```python
from build123d import *

# Parameters (mm, degrees)
SKETCH1_W              = 20
SKETCH1_H              = 35
SKETCH1_R              = 5
SKETCH1_R_2            = 1.1
BOSS_EXTRUDE1_DEPTH    = 13
SKETCH5_W              = 16
SKETCH5_H              = 31
CUT_EXTRUDE1_DEPTH     = 11
CUT_EXTRUDE2_REACH     = 40.652
SKETCH7_R              = 1.5
BOSS_EXTRUDE3_DEPTH    = 13
SKETCH11_R             = 3.25
CUT_EXTRUDE4_DEPTH     = 12
CUT_EXTRUDE5_START     = 12
CUT_EXTRUDE5_OUTLINE_R = 1.75
CUT_EXTRUDE5_DEPTH     = 1


# Read off the part's stored shape, not the designer's step: Cut-Extrude5
with BuildPart() as part:
    # Sketch1 → Boss-Extrude1 (new body)
    with BuildSketch(Plane(origin=(0, 0, 0), x_dir=(1, 0, 0), z_dir=(0, 1, 0))):
        with Locations((0, -7.840328725)):
            Rectangle(SKETCH1_W, SKETCH1_H)
        with Locations(Location((0, 0, 0), (0, 0, 90))):
            Circle(SKETCH1_R, mode=Mode.SUBTRACT)
        with Locations(Location((6.35, 0, 0), (0, 0, 90))):
            Circle(SKETCH1_R_2, mode=Mode.SUBTRACT)
    extrude(amount=BOSS_EXTRUDE1_DEPTH)

    # Sketch5 → Cut-Extrude1 (cut)
    with BuildSketch(Plane(origin=(0, 13, 0), x_dir=(1, 0, 0), z_dir=(0, 1, 0))):
        with Locations((0, -7.840328725)):
            Rectangle(SKETCH5_W, SKETCH5_H)
    extrude(amount=-CUT_EXTRUDE1_DEPTH, mode=Mode.SUBTRACT)

    # Sketch7 → Cut-Extrude2 (cut, up to next)
    with BuildSketch(Plane.XY.offset(25.340328725), mode=Mode.PRIVATE) as cut_extrude2_sk1:
        with Locations((0, 7)):
            Circle(SKETCH7_R)
    cut_extrude2_tool1 = extrude(cut_extrude2_sk1.sketch, amount=-CUT_EXTRUDE2_REACH, mode=Mode.PRIVATE) & part.part
    add(cut_extrude2_tool1.solids().sort_by_distance((0, 7, 25.340329))[0], mode=Mode.SUBTRACT)

    # Sketch9 → Boss-Extrude3 (add, through all)
    with BuildSketch(Plane(origin=(0, 13, 0), x_dir=(1, 0, 0), z_dir=(0, 1, 0))):
        with BuildLine():
            Line((-14, 7.159671275), (-10, 7.159671275))
            Line((-10, 7.159671275), (-10, -2.840328725))
            Line((-10, -2.840328725), (-14, -2.840328725))
            ThreePointArc((-14, -2.840328725), (-19, 2.159671275), (-14, 7.159671275))
        make_face()
        with BuildLine():
            Line((-14, -7.804369497), (-10, -7.804369497))
            Line((-10, -7.804369497), (-10, -17.804369497))
            Line((-10, -17.804369497), (-14, -17.804369497))
            ThreePointArc((-14, -17.804369497), (-19, -12.804369497), (-14, -7.804369497))
        make_face()
        with BuildLine():
            Line((10, -7.804369497), (10, -17.804369497))
            Line((10, -17.804369497), (14, -17.804369497))
            ThreePointArc((14, -17.804369497), (19, -12.804369497), (14, -7.804369497))
            Line((14, -7.804369497), (10, -7.804369497))
        make_face()
        with BuildLine():
            Line((10, 7.159671275), (10, -2.840328725))
            Line((10, -2.840328725), (14, -2.840328725))
            ThreePointArc((14, -2.840328725), (19, 2.159671275), (14, 7.159671275))
            Line((14, 7.159671275), (10, 7.159671275))
        make_face()
    extrude(amount=-BOSS_EXTRUDE3_DEPTH)

    # Sketch11 → Cut-Extrude4 (cut)
    with BuildSketch(Plane.XZ):
        with Locations(Location((-14, 12.800328725, 0), (0, 0, 270))):
            Circle(SKETCH11_R)
        with Locations(Location((-14, -2.159671275, 0), (0, 0, 270))):
            Circle(SKETCH11_R)
        with Locations(Location((14, 12.800328725, 0), (0, 0, 270))):
            Circle(SKETCH11_R)
        with Locations(Location((14, -2.159671275, 0), (0, 0, 270))):
            Circle(SKETCH11_R)
    extrude(amount=-CUT_EXTRUDE4_DEPTH, mode=Mode.SUBTRACT)

    # Cut-Extrude5 outline → Cut-Extrude5 (cut)
    with BuildSketch(Plane(origin=(0, 0, 0), x_dir=(1, 0, 0), z_dir=(0, 1, 0)).offset(CUT_EXTRUDE5_START)):
        with Locations((-14, 2.159671275)):
            Circle(CUT_EXTRUDE5_OUTLINE_R)
        with Locations((14, -12.800328725)):
            Circle(CUT_EXTRUDE5_OUTLINE_R)
        with Locations((14, 2.159671275)):
            Circle(CUT_EXTRUDE5_OUTLINE_R)
        with Locations((-14, -12.800328725)):
            Circle(CUT_EXTRUDE5_OUTLINE_R)
    extrude(amount=CUT_EXTRUDE5_DEPTH, mode=Mode.SUBTRACT)


solid = part.part
```
The model under review builds one solid part; all positions refer to its coordinate system, in mm. A direction names the side the tool comes from. Coordinates: 2 decimals unless noted, no trailing zeros. Order: outer loops, then holes, each group sorted by start corner. A loop starts at its lowest first (then second) coordinate and runs counter-clockwise, first axis right, second up. Notation, with made-up numbers: M 11,81 L 67,81 A26 cw 67,106 Z; hole C -15,81 d3. An arc over 180 degrees is marked long. One line per question, with ' | ' between items.
(1) Add section B-B, the plane y = 7. State how many separate pieces and enclosed holes the cut face has, then the cut area to 3 significant figures.
Geometry results:
separate pieces: 1 | enclosed holes: 4 | area: 382 mm²
(2) For probe 1 along X at (y, z) = (3.5, 13); probe 2 along Z at (x, y) = (-14, 12.6); probe 3 along X at (y, z) = (2.5, 20.5), list the stretches that pass through material, from the lowest coordinate up. Write a range as from..to.
Geometry results:
probe 1: x = -19..-17.24, -10.76..-8, 8..10.76, 17.24..19 | probe 2: z = -7.16..-3.91, -0.41..2.84, 7.8..11.05, 14.55..17.8 | probe 3: x = -10..-8, 8..10
(3) Add section A-A, the plane x = 0. Write out the cut boundary in (y, z), then the cut area to 3 significant figures.
Geometry results:
outline: M 0,-9.66 L 13,-9.66 L 13,-7.66 L 2,-7.66 L 2,-5 L 0,-5 Z; M 0,5 L 2,5 L 2,23.34 L 5.5,23.34 L 5.5,25.34 L 0,25.34 Z; M 8.5,23.34 L 13,23.34 L 13,25.34 L 8.5,25.34 Z | area: 88.0 mm²
(4) Add section C-C, the plane z = 2. Write out the cut boundary in (x, y).
Geometry results:
outline: M -16.77,0 L -4.58,0 L -4.58,2 L -8,2 L -8,13 L -16.77,13 Z; M 4.58,0 L 16.77,0 L 16.77,13 L 8,13 L 8,2 L 4.58,2 Z
(5) Machinability: for faces 4 (the face through (12, 7, 17.804)), 5 (the face through (10, 6, 5)), 6 (the face through (13, 12, -4)), 7 (the face through (12, 7, -7.16)), which of the approach directions +Z, -Z, +X, -X, +Y, -Y give a long, thin tool a straight path to every point of the face, cutting with its end or side? Answer none if there is none.
Geometry results:
face 4: +Z, +X, +Y, -Y | face 5: +X, +Y, -Y | face 6: -Y | face 7: -Z, +X, +Y, -Y
(6) Add section D-D, the plane x = 6.35. Write out the cut boundary in (y, z).
Geometry results:
outline: M 0,-9.66 L 13,-9.66 L 13,-7.66 L 2,-7.66 L 2,-1.1 L 0,-1.1 Z; M 0,1.1 L 2,1.1 L 2,23.34 L 13,23.34 L 13,25.34 L 0,25.34 Z
(7) The part is to be moulded in two halves that separate along Z. For faces 1 (the face through (0, 5, 25.34)), 2 (the face through (-15, 12, -4)), 3 (the face through (8.2, 13, 3.7)), say which applies: +Z half, -Z half, draft (parallel to the pull), parting line (faces both ways), or undercut.
Geometry results:
face 1: +Z half | face 2: undercut | face 3: draft
(8) Insertion check: pin 1 (2.5 mm diameter, centred on y = 3.5, z = 23, fed in from +X); pin 2 (3 mm diameter, centred on x = 13, z = 14, fed in from -Y); pin 3 (5.5 mm diameter, centred on y = 8.5, z = 3, fed in from -X). Each pin has a flat end and moves straight along its axis. Give the tip position at first contact, or say it passes through.
Geometry results:
pin 1: stops at x = 10 | pin 2: stops at y = 12 | pin 3: stops at x = -18.38
